Autodesk Inventor part; units mm, degrees
ref_plane "YZ Plane" through (0, 0, 0) normal (1, 0, 0) x (0, 1, 0)
ref_plane "XZ Plane" through (0, 0, 0) normal (0, 1, 0) x (-1, 0, 0)
ref_plane "XY Plane" through (0, 0, 0) normal (0, 0, 1) x (1, 0, 0)
sketch "Esquisse1" plane through (0, 0, 0) normal (0, 1, 0) x (-1, 0, 0)
  line L0 (53.1259, 14.235) -> (0, 0)
  line L1 (47.9495, 33.5536) -> (53.1259, 14.235)
  line L2 (-45, 0) -> (-45, 20)
  line L3 (-45, 0) -> (0, 0)
  line L4 (-45, 20) -> (-2.633, 20)
  line L5 (47.9495, 33.5536) -> (-2.633, 20)
  dimension "d1" = 20
  dimension "d4" = 20
  dimension "d7" = 45
  dimension "d9" = 55
  dimension "d11" = 15
extrude "Extrusion1" add sketch "Esquisse1" along normal blind 35
sketch "Esquisse3" plane through (2.633, 0, 20) normal (0, 0, 1) x (1, 0, 0)
  line L0 (0, 0) -> (0, 35)
  line L1 (-65, 20) -> (0, 20)
  line L2 (0, 20) -> (0, 15)
  line L3 (0, 15) -> (-65, 15)
  line L4 (-65, 15) -> (-65, 20)
  line L5 (-2.633, 35) -> (-55.759, 35)
  point P0 (-2.633, 0)
  point P1 (0, 20)
  dimension "d14" = 5
  dimension "d15" = 65
  dimension "d16" = 15
extrude "Extrusion2" cut sketch "Esquisse3" along normal through all both and the other way through all
equation "\"d1\" = d4"
properties part number "Equerre_gauche"
The listing builds one solid part. Answer for the finished solid, in the listing's coordinates (mm). A direction names the side the tool comes from. Coordinates: 2 decimals unless noted, no trailing zeros. Loops run counter-clockwise (first coordinate to the right, second up) from the corner with the lowest first, then second, coordinate; pieces in that order, holes last. Notation, with made-up numbers: (9.25, -8) -> (20.25, -8) arc R16 cw to (20.25, 18) -> close; hole circle Ø11 at (54, -29). An arc over 180 degrees is marked (long way). Write item = value, one per line. Start each with the question number.
1) The mould has two halves that part along Y. Classify faces 1 (the face through (-23.01, 7.4, 26.87)), 2 (the face through (-3, 0, 13)), 3 (the face through (-3, 35, 13)), 4 (the face through (-26, 20, 17)): released by +Y, released by -Y, zero draft, split by the parting line, or undercut.
2) A cutting plane is placed at B-B (x = -45.5). Give the vertices of the cut face in (y, z).
3) Straight lines are drawn through the part: line 1 (Y direction, x = 2, z = 6.5); line 2 (X direction, y = 19, z = 5); line 3 (Z direction, x = 14.5, y = 33). For each, find the intervals that lie inside material, in ascending order. Write a range as from..to.
4) A cutting plane is placed at A-A (z = 27). Give the vertices of the cut face in (x, y), then the cut area to 3 significant figures.
5) A cutting plane is placed at C-C (y = 32). Give the vertices of the cut face in (x, z) (1 decimal).
6) A cutting plane is placed at D-D (x = 10.5). Give the vertices of the cut face in (y, z), then the cut area to 3 significant figures.
7) A tool of negligible diameter and unlimited length cuts with its end or side. For faces 5 (the face through (-50.5, 27.4, 24.03)), 6 (the face through (24, 17, 20)), 7 (the face through (-25, 15, 17)), from which of +Z, -Z, +X, -X, +Y, -Y can it reach the whole face along a straight path? Write none if from no direction.
8) Given pin 1 Ø8 at (y, z) = (14, 25.5) entering from -X; pin 2 Ø1.5 at (y, z) = (18, 11) entering from -X; pin 3 Ø3 at (x, y) = (2.5, 20.5) entering from +Z, each flat-ended and moving along its own axis, determine where each tip first touches the part or whether it passes through.
Responses:
q1.face_1 = zero draft
q1.face_2 = released by -Y
q1.face_3 = released by +Y
q1.face_4 = undercut
q2.outline = (0, 12.19) -> (15, 12.19) -> (15, 32.9) -> (0, 32.9) -> close; (20, 12.19) -> (35, 12.19) -> (35, 32.9) -> (20, 32.9) -> close
q3.line_1 = 0..15, 20..35
q3.line_2 = 2.63..45
q3.line_3 = 0..20
q4.outline = (-49.71, 0) -> (-23.49, 0) -> (-23.49, 15) -> (-49.71, 15) -> close; (-49.71, 20) -> (-23.49, 20) -> (-23.49, 35) -> (-49.71, 35) -> close
q4.area = 786 mm²
q5.outline = (-53.1, 14.2) -> (0, 0) -> (45, 0) -> (45, 20) -> (2.6, 20) -> (-47.9, 33.6) -> close
q6.outline = (0, 0) -> (35, 0) -> (35, 20) -> (0, 20) -> close
q6.area = 700 mm²
q7.face_5 = +Z, -X, +Y, -Y
q7.face_6 = +Z, +X, +Y, -Y
q7.face_7 = +Z, -Z, -X
q8.pin_1 = -51.18
q8.pin_2 = 2.63
q8.pin_3 = 20.44
